CAD build for the part. Positions are in the model's coordinates, mm. A direction names the side the tool comes from. Give positions to 0.01 mm unless a question says otherwise; leave off trailing zeros. Write each loop counter-clockwise with the first axis right and the second up, starting at its lowest first coordinate (ties: lowest second). Pieces come first, ordered by that corner, then holes. Notation, with made-up numbers: (73, 36) -> (110, 36) arc R29 ccw to (110, 69) -> close; hole circle Ø2 at (74.25, 66.25). An arc over 180 degrees is marked (long way). Use one line per item in the form item = value. Start each with the question number.
from build123d import *

# Parameters (mm, degrees)
F0_R     = 73.025
F1_DEPTH = 69.85
F3_DEPTH = 60.96
F4_R     = 12.7
F5_R     = 10.16


with BuildPart() as f1:
    # F0 (on Front) → F1 (new body)
    with BuildSketch(Plane.XZ):
        Circle(F0_R)
    extrude(amount=F1_DEPTH)

    # F2 (on face) → F3 (cut)
    with BuildSketch(Plane.XZ.offset(69.85)):
        with BuildLine():
            Line((-9.6547204396, -59.5473928752), (-9.6547204396, 59.5473928752))
            ThreePointArc((-9.6547204396, 59.5473928752), (-60.325, 0), (-9.6547204396, -59.5473928752))
        make_face()
        with BuildLine():
            ThreePointArc((9.652, -59.5478338901), (45.9421512611, -39.0950682631), (60.325, 0))
            ThreePointArc((60.325, 0), (45.9421512611, 39.0950682631), (9.652, 59.5478338901))
            Line((9.652, 59.5478338901), (9.652, -59.5478338901))
        make_face()
    extrude(amount=-F3_DEPTH, mode=Mode.SUBTRACT)

    # F4
    f4_edges = [f1.edges().sort_by_distance(p)[0] for p in [
        (9.652, -39.37, 59.547834),
        (-9.65472, -39.37, 59.547393),
        (9.652, -39.37, -59.547834),
        (-9.65472, -39.37, -59.547393),
    ]]
    fillet(f4_edges, radius=F4_R)

    # F5
    f5_edges = [f1.edges().sort_by_distance(p)[0] for p in [
        (-73.025, 0, 0),
    ]]
    fillet(f5_edges, radius=F5_R)


solid = f1.part
1) Cut at A-A (y = -60). Give the cut face in (x, z) (3 decimals), and give its area (3 significant figures).
2) 3-axis set-ups, long thin cutter, end or side, ignore diameter. For faces 1 (the face through (-9.655, -40, -1)), 2 (the face through (0, -69.85, 6)): which of +Z, -Z, +X, -X, +Y, -Y reach the whole face in a straight line?
3) Wall check: line 1 along X through (y, z) = (-38.5, -0.5); line 2 along X through (y, z) = (-9, 27); line 3 along Y through (x, z) = (-54.5, -2.5). Give the ranges that are in metal, low to high. Write a range as from..to.
4) Two-plate mould, pull along Z, no slides. Class faces 3 (the face through (-15.657, -38.943, 52.843)), 4 (the face through (-1, 0, 1)), 5 (the face through (69.653, -39.587, 21.935)): released by +Z, released by -Z, zero draft, split by the parting line, or undercut.
5) Pin check, flat tips, straight feed: pin 1 (1 mm diameter, centred on y = -33.5, z = -27.5, fed in from +X); pin 2 (15 mm diameter, centred on x = 38, z = 22.5, fed in from -Y); pin 3 (1.5 mm diameter, centred on x = -1.5, y = -21.5, fed in from -Z). Stop position of each tip, or through.
Final values:
q1.outline = circle Ø146.05 at (0, 0); hole (-28.316, -53.266) arc R12.7 ccw to (-9.655, -42.052) -> (-9.655, 42.052) arc R12.7 ccw to (-28.316, 53.266) arc R60.325 ccw to start; hole (9.652, -42.054) arc R12.7 ccw to (28.313, -53.268) arc R60.325 ccw to (28.313, 53.268) arc R12.7 ccw to (9.652, 42.054) -> close
q1.area = 7,960 mm^2
q2.face_1 = -Y
q2.face_2 = +Z, -Z, +X, -X, -Y
q3.line_1 = -73.02..-60.32, -9.65..9.65, 60.32..73.02
q3.line_2 = -67.78..-53.95, -9.65..9.65, 53.95..67.78
q3.line_3 = -8.89..0
q4.face_3 = undercut
q4.face_4 = zero draft
q4.face_5 = split by the parting line
q5.pin_1 = 67.85
q5.pin_2 = -8.89
q5.pin_3 = -73.02
